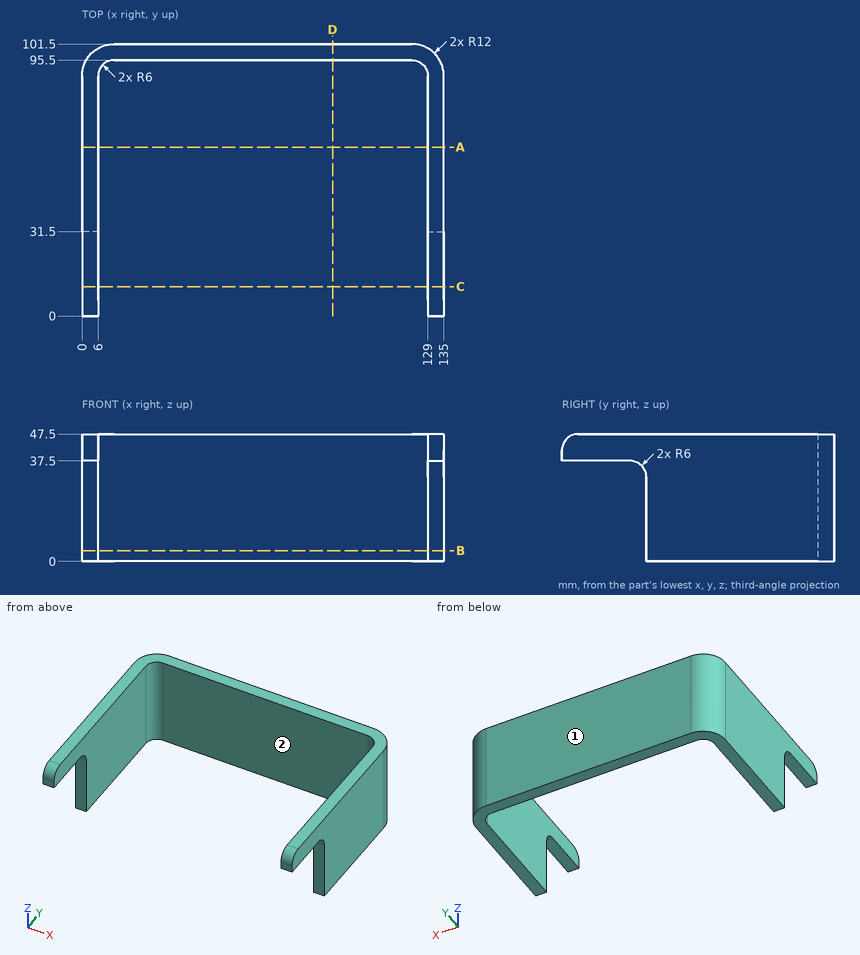
Study the drawing (mm; zero at the part's minimum x, y, z) and answer. A direction names the side the tool comes from. Round coordinates to 2 decimals unless told otherwise and drop trailing zeros. Loops run counter-clockwise (first coordinate to the right, second up) from the corner with the lowest first, then second, coordinate; pieces in that order, holes last.
Q1. Section B-B, the plane z = 4 is taken. Determine the outline of the cut face in (x, y), then the cut area to 3 significant figures.
Q2. Section C-C, the plane y = 11 is taken. Determine the outline of the cut face in (x, z), then the cut area to 3 significant figures.
Q3. Given pin 1 Ø3 at (x, y) = (131, 18) entering from -Z; pin 2 Ø6.5 at (x, z) = (3, 19) entering from -Y; pin 3 Ø12 at (x, y) = (65, 88) entering from +Z, each flat-ended and moving along its own axis, determine where each tip first touches the part or whether it passes through.
Q4. Which of the six approach directions +Z, -Z, +X, -X, +Y, -Y give full straight-line access (tool end or side, diameter ignored) to the marked faces 1 and 2?
Q5. Find the intervals of material crossed by line 1 (X direction, y = 88.5, z = 9.5); line 2 (Y direction, x = 95.5, z = 22.5); line 3 (Y direction, x = 8, z = 35.5), in increasing order.
Q6. Section D-D, the plane x = 93.5 is taken. Determine the outline of the cut face in (y, z).
Q7. Section A-A, the plane y = 63 is taken. Determine the outline of the cut face in (x, z).
Completed:
1. outline: (0, 31.5) - (6, 31.5) - (6, 89.5) arc R6 cw to (12, 95.5) - (123, 95.5) arc R6 cw to (129, 89.5) - (129, 31.5) - (135, 31.5) - (135, 89.5) arc R12 ccw to (123, 101.5) - (12, 101.5) arc R12 ccw to (0, 89.5) - close
1. area: 1,530 mm2
2. outline: (0, 37.5) - (6, 37.5) - (6, 47.5) - (0, 47.5) - close; (129, 37.5) - (135, 37.5) - (135, 47.5) - (129, 47.5) - close
2. area: 120 mm2
3. pin 1: stops at z = 37.5
3. pin 2: stops at y = 31.5
3. pin 3: passes through
4. face 1: +Z, -Z, +X, -X, +Y
4. face 2: +Z, -Z, -Y
5. line 1: x = 0 to 6, 129 to 135
5. line 2: y = 95.5 to 101.5
5. line 3: y = 93.97 to 100.81
6. outline: (95.5, 0) - (101.5, 0) - (101.5, 47.5) - (95.5, 47.5) - close
7. outline: (0, 0) - (6, 0) - (6, 47.5) - (0, 47.5) - close; (129, 0) - (135, 0) - (135, 47.5) - (129, 47.5) - close
